from build123d import *

# Parameters (mm, degrees)
CROQUIS1_W              = 404
CROQUIS1_H              = 400
SALIENTE_EXTRUIR1_DEPTH = 2
CROQUIS3_W              = 157
CROQUIS3_H              = 90
CORTAR_EXTRUIR2_DEPTH   = 2
REDONDEO1_R             = 5
CORTAR_EXTRUIR3_DEPTH   = 2
REDONDEO2_R             = 20
CROQUIS6_R              = 1.55
CORTAR_EXTRUIR5_DEPTH   = 2
CROQUIS7_R              = 1.55
CORTAR_EXTRUIR6_DEPTH   = 2
CROQUIS8_W              = 20
CROQUIS8_H              = 100
SALIENTE_EXTRUIR2_DEPTH = 2
REDONDEO3_R             = 10
CROQUIS9_R              = 1.55
CORTAR_EXTRUIR7_DEPTH   = 2
CROQUIS10_OUTSIDE_W     = 519.704
CROQUIS10_OUTSIDE_H     = 515.704
CORTAR_EXTRUIR8_DEPTH   = 10
CROQUIS11_W             = 245
CROQUIS11_H             = 1
CORTAR_EXTRUIR9_DEPTH   = 2
CROQUIS12_W             = 1
CROQUIS12_H             = 308
SALIENTE_EXTRUIR3_DEPTH = 2


with BuildPart() as part:
    # Croquis1 → Saliente-Extruir1 (new body)
    with BuildSketch(Plane(origin=(0, 0, 0), x_dir=(1, 0, 0), z_dir=(0, 1, 0))):
        with Locations((202, 200)):
            Rectangle(CROQUIS1_W, CROQUIS1_H)
    extrude(amount=SALIENTE_EXTRUIR1_DEPTH)

    # Croquis3 → Cortar-Extruir2 (cut)
    with BuildSketch(Plane.XZ):
        with Locations((78.5, -355)):
            Rectangle(CROQUIS3_W, CROQUIS3_H)
    extrude(amount=-CORTAR_EXTRUIR2_DEPTH, mode=Mode.SUBTRACT)

    # Redondeo1
    redondeo1_edges = [part.edges().sort_by_distance(p)[0] for p in [
        (157, 1, -310),
    ]]
    fillet(redondeo1_edges, radius=REDONDEO1_R)

    # Croquis4 → Cortar-Extruir3 (cut)
    with BuildSketch(Plane.XZ):
        Polygon((30, -20), (364, -20), (364, -233.661541009), (364, -370), (182, -370), (182, -285), (30, -285), align=None)
    extrude(amount=-CORTAR_EXTRUIR3_DEPTH, mode=Mode.SUBTRACT)

    # Redondeo2
    redondeo2_edges = [part.edges().sort_by_distance(p)[0] for p in [
        (30, 1, -285),
        (30, 1, -20),
        (364, 1, -20),
        (364, 1, -370),
        (182, 1, -370),
        (182, 1, -285),
    ]]
    fillet(redondeo2_edges, radius=REDONDEO2_R)

    # Croquis6 → Cortar-Extruir5 (cut)
    with BuildSketch(Plane.XZ):
        with Locations(Location((75, -14, 0), (0, 0, 270))):
            Circle(CROQUIS6_R)
        with Locations(Location((275, -14, 0), (0, 0, 270))):
            Circle(CROQUIS6_R)
        with Locations(Location((273, -376, 0), (0, 0, 270))):
            Circle(CROQUIS6_R)
        with Locations(Location((106, -291, 0), (0, 0, 270))):
            Circle(CROQUIS6_R)
        with Locations(Location((24, -152.5, 0), (0, 0, 270))):
            Circle(CROQUIS6_R)
        with Locations(Location((370, -152.5, 0), (0, 0, 270))):
            Circle(CROQUIS6_R)
    extrude(amount=-CORTAR_EXTRUIR5_DEPTH, mode=Mode.SUBTRACT)

    # Croquis7 → Cortar-Extruir6 (cut)
    with BuildSketch(Plane.XZ):
        with Locations(Location((394.25, -25, 0), (0, 0, 270))):
            Circle(CROQUIS7_R)
        with Locations(Location((394.25, -39, 0), (0, 0, 270))):
            Circle(CROQUIS7_R)
        with Locations(Location((394.25, -375, 0), (0, 0, 270))):
            Circle(CROQUIS7_R)
        with Locations(Location((394.25, -361, 0), (0, 0, 270))):
            Circle(CROQUIS7_R)
    extrude(amount=-CORTAR_EXTRUIR6_DEPTH, mode=Mode.SUBTRACT)

    # Croquis8 → Saliente-Extruir2 (add)
    with BuildSketch(Plane.XZ):
        with Locations((40, -155)):
            Rectangle(CROQUIS8_W, CROQUIS8_H)
    extrude(amount=-SALIENTE_EXTRUIR2_DEPTH)

    # Redondeo3
    redondeo3_edges = [part.edges().sort_by_distance(p)[0] for p in [
        (30, 1, -205),
        (30, 1, -105),
    ]]
    fillet(redondeo3_edges, radius=REDONDEO3_R)
    redondeo3_2_edges = [part.edges().sort_by_distance(p)[0] for p in [
        (50, 1, -205),
        (50, 1, -105),
    ]]
    fillet(redondeo3_2_edges, radius=REDONDEO3_R - 0.0001)  # a hair under: the kernel refuses the full size

    # Croquis9 → Cortar-Extruir7 (cut)
    with BuildSketch(Plane.XZ):
        with Locations(Location((42, -115, 0), (0, 0, 270))):
            Circle(CROQUIS9_R)
        with Locations(Location((42, -195, 0), (0, 0, 270))):
            Circle(CROQUIS9_R)
    extrude(amount=-CORTAR_EXTRUIR7_DEPTH, mode=Mode.SUBTRACT)

    # Croquis10 outside → Cortar-Extruir8 (cut)
    with BuildSketch(Plane.XZ):
        with Locations((202, -200)):
            Rectangle(CROQUIS10_OUTSIDE_W, CROQUIS10_OUTSIDE_H)
        with BuildLine():
            Line((1, -309), (152, -309))
            ThreePointArc((152, -309), (156.242640687, -310.757359313), (158, -315))
            Line((158, -315), (158, -399))
            Line((158, -399), (403, -399))
            Line((403, -399), (403, -1))
            Line((403, -1), (1, -1))
            Line((1, -1), (1, -309))
        make_face(mode=Mode.SUBTRACT)
    extrude(amount=-CORTAR_EXTRUIR8_DEPTH, mode=Mode.SUBTRACT)

    # Croquis11 → Cortar-Extruir9 (cut)
    with BuildSketch(Plane.XZ):
        with Locations((280.5, -398.5)):
            Rectangle(CROQUIS11_W, CROQUIS11_H)
    extrude(amount=-CORTAR_EXTRUIR9_DEPTH, mode=Mode.SUBTRACT)

    # Croquis12 → Saliente-Extruir3 (add)
    with BuildSketch(Plane.XZ):
        with Locations((0.5, -155)):
            Rectangle(CROQUIS12_W, CROQUIS12_H)
    extrude(amount=-SALIENTE_EXTRUIR3_DEPTH)


solid = part.part
Geometry: final body of the model. Coordinates: model frame, mm. A direction names the side the tool comes from. Coordinates: 2 decimals unless noted, no trailing zeros. Loops run counter-clockwise (first coordinate to the right, second up) from the corner with the lowest first, then second, coordinate; pieces in that order, holes last. Notation, with made-up numbers: (29.25, -20) - (69.25, -20) arc R27 ccw to (69.25, 11) - close; hole circle Ø9 at (-21, 30.5). An arc over 180 degrees is marked (long way). Put each result on its own line as item: value. Start each with the question number.
Q1. Cut plane C-C, the plane z = -333. Return loops of the section in (x, y), and give its area (3 significant figures).
Q2. Line query: line 1 (X direction, y = 1.15, z = -152.5); line 2 (X direction, y = 0.6, z = -39); line 3 (X direction, y = 0.95, z = -14). Output: solid intervals per line, ascending.
Q3. Pull-direction query (Z, two-part tool) for faces 3 (the flat face through (126, 2, -287)), 4 (the cylindrical face through (188.014, 1.014, -364.297)); classes: released by +Z, released by -Z, zero draft, split by the parting line, or undercut.
Q4. Cut plane B-B, the plane y = 0.75. Give the number of separate pieces and of enclosed holes in the cut face, and give its area (3 significant figures).
Q5. Set-up query: faces 1 (the flat face through (126, 0, -287)), 2 (the cylindrical face through (176.297, 1.014, -291.014)). Return all of +Z, -Z, +X, -X, +Y, -Y with unobstructed straight access to the full face (end or side cutting, diameter ignored); none if empty.
Q6. Cut plane A-A, the plane z = -68.5. Return loops of the section in (x, y), and give its area (3 significant figures).
Filled sheet:
1. outline: (158, 0) - (182, 0) - (182, 2) - (158, 2) - close; (364, 0) - (403, 0) - (403, 2) - (364, 2) - close
1. area: 126 mm²
2. line 1: 0 to 22.45, 25.55 to 50, 364 to 368.45, 371.55 to 403
2. line 2: 0 to 30.03, 363.97 to 392.7, 395.8 to 403
2. line 3: 0 to 73.45, 76.55 to 273.45, 276.55 to 403
3. face 3: zero draft
3. face 4: undercut
4. separate pieces: 1
4. enclosed holes: 13
4. area: 44,200 mm²
5. face 1: +Z, -Z, +X, -X, -Y
5. face 2: +Y, -Y
6. outline: (0, 0) - (30, 0) - (30, 2) - (0, 2) - close; (364, 0) - (403, 0) - (403, 2) - (364, 2) - close
6. area: 138 mm²
